```python
from build123d import *

# Parameters (mm, degrees)
F0_W          = 25
F0_H          = 52
F0_R          = 1
F1_DEPTH      = 2
F0_W_2        = 51
F0_H_2        = 170
F0_R_2        = 1.5
F2_DEPTH      = 3
F3_W          = 51
F3_H          = 170
F4_DEPTH      = 4
F5_R          = 1.5
F5_R_2        = 1
F6_DEPTH      = 5
F6_DEPTH_BACK = 3
F7_R          = 1.5
F7_R_2        = 1
F8_DEPTH      = 7


with BuildPart() as f1:
    # F0 (on Top) → F1 (new body)
    with BuildSketch(Plane.XY):
        with Locations((12.5, -86)):
            Rectangle(F0_W, F0_H)
        with Locations((12.5, -69.3)):
            Circle(F0_R, mode=Mode.SUBTRACT)
        with Locations((12.5, 26)):
            Rectangle(F0_W, F0_H)
        with Locations((12.5, 9.3)):
            Circle(F0_R, mode=Mode.SUBTRACT)
    extrude(amount=F1_DEPTH)

    # F0 (on Top) → F2 (join)
    with BuildSketch(Plane.XY):
        with Locations((12.5, -30)):
            Rectangle(F0_W_2, F0_H_2)
        with Locations((12.5, -86)):
            Rectangle(F0_W, F0_H, mode=Mode.SUBTRACT)
        with Locations((12.5, -56.36)):
            Circle(F0_R_2, mode=Mode.SUBTRACT)
        with Locations((12.5, -31.5)):
            Circle(F0_R_2, mode=Mode.SUBTRACT)
        with Locations((12.5, -3.64)):
            Circle(F0_R_2, mode=Mode.SUBTRACT)
        with Locations((12.5, 26)):
            Rectangle(F0_W, F0_H, mode=Mode.SUBTRACT)
        with Locations((12.5, -86)):
            Rectangle(F0_W, F0_H)
        with Locations((12.5, -69.3)):
            Circle(F0_R, mode=Mode.SUBTRACT)
        with Locations((12.5, 26)):
            Rectangle(F0_W, F0_H)
        with Locations((12.5, 9.3)):
            Circle(F0_R, mode=Mode.SUBTRACT)
    extrude(amount=-F2_DEPTH)

    # F3 (on face) → F4 (join)
    with BuildSketch(Plane.XY):
        with Locations((12.5, -30)):
            Rectangle(F3_W, F3_H)
        Polygon((-10, -112), (-10, 52), (0, 52), (25, 52), (35, 52), (35, -112), (25, -112), (0, -112), align=None, mode=Mode.SUBTRACT)
    extrude(amount=F4_DEPTH)

    # F5 (on face) → F6 (join, two sides)
    with BuildSketch(Plane.XY) as f6_sk:
        with Locations((12.5, -3.64)):
            Circle(F5_R)
        with Locations((12.5, -3.64)):
            Circle(F5_R_2, mode=Mode.SUBTRACT)
        with Locations((12.5, -31.5)):
            Circle(F5_R)
        with Locations((12.5, -31.5)):
            Circle(F5_R_2, mode=Mode.SUBTRACT)
        with Locations((12.5, -56.36)):
            Circle(F5_R)
        with Locations((12.5, -56.36)):
            Circle(F5_R_2, mode=Mode.SUBTRACT)
    extrude(amount=F6_DEPTH)
    extrude(f6_sk.sketch, amount=-F6_DEPTH_BACK)

    # F7 (on face) → F8 (cut)
    with BuildSketch(Plane.XY.offset(5)):
        with Locations((12.5, -31.5)):
            Circle(F7_R)
        with Locations((12.5, -31.5)):
            Circle(F7_R_2, mode=Mode.SUBTRACT)
    extrude(amount=-F8_DEPTH, mode=Mode.SUBTRACT)


solid = f1.part
```
Here's how the part is built. I have some questions about the finished solid (model axes, mm). A direction names the side the tool comes from. Coordinates: 2 decimals unless noted, no trailing zeros. Order: outer loops, then holes, each group sorted by start corner. A loop starts at its lowest first (then second) coordinate and runs counter-clockwise, first axis right, second up.
1) Imagine slicing it at B-B on y = -47. List the corners of the cut face in (x, z) for me, and give its area (3 significant figures).
2) We'd pull the mould along Y, two halves only. Please class faces 1 (the face through (12, 55, 0)), 2 (the face through (12, -86, 2)), 3 (the face through (38, -31, 0)): +Y half, -Y half, draft (parallel to the pull), parting line (faces both ways), or undercut.
3) Will these pins go through, and if not, where does the flat tip stop? pin 1 (22.5 mm diameter, centred on x = 15.5, y = -21, fed in from +Z); pin 2 (1.5 mm diameter, centred on x = 4, y = -59.5, fed in from +Z); pin 3 (1.5 mm diameter, centred on x = 12.5, y = -32, fed in from +Z).
4) Imagine slicing it at C-C on y = 42. List the corners of the cut face in (x, z) for me.
5) I need wall thicknesses on line 1 (Y direction, x = 12.5, z = -2.05); line 2 (X direction, y = 11.5, z = 0.25); line 3 (Y direction, x = 14.5, z = 3.25). Which ranges of each line are inside material? Lowest first, please.
6) Which directions (+Z, -Z, +X, -X, +Y, -Y) give clear straight access to the entire face, cutting with the end or side of a thin tool? Please do faces 4 (the face through (12, -115, 0)), 5 (the face through (12.305, -54.873, 2.465)).
7) Imagine slicing it at A-A on x = 33. List the corners of the cut face in (y, z) for me, and give its area (3 significant figures).
Response values:
1. outline: (-13, -3) - (38, -3) - (38, 4) - (35, 4) - (35, 0) - (-10, 0) - (-10, 4) - (-13, 4) - close
1. area: 177 mm2
2. face 1: +Y half
2. face 2: undercut
2. face 3: draft
3. pin 1: stops at z = 0
3. pin 2: stops at z = 2
3. pin 3: stops at z = -2
4. outline: (-13, -3) - (38, -3) - (38, 4) - (35, 4) - (35, 0) - (25, 0) - (25, 2) - (0, 2) - (0, 0) - (-10, 0) - (-10, 4) - (-13, 4) - close
5. line 1: y = -115 to -70.3, -68.3 to -57.36, -55.36 to -32.5, -30.5 to -4.64, -2.64 to 8.3, 10.3 to 55
5. line 2: x = -13 to -10, 0 to 25, 35 to 38
5. line 3: y = -115 to -112, 52 to 55
6. face 4: +Z, -Z, +X, -X, -Y
6. face 5: +Z
7. outline: (-115, -3) - (55, -3) - (55, 4) - (52, 4) - (52, 0) - (-112, 0) - (-112, 4) - (-115, 4) - close
7. area: 534 mm2
